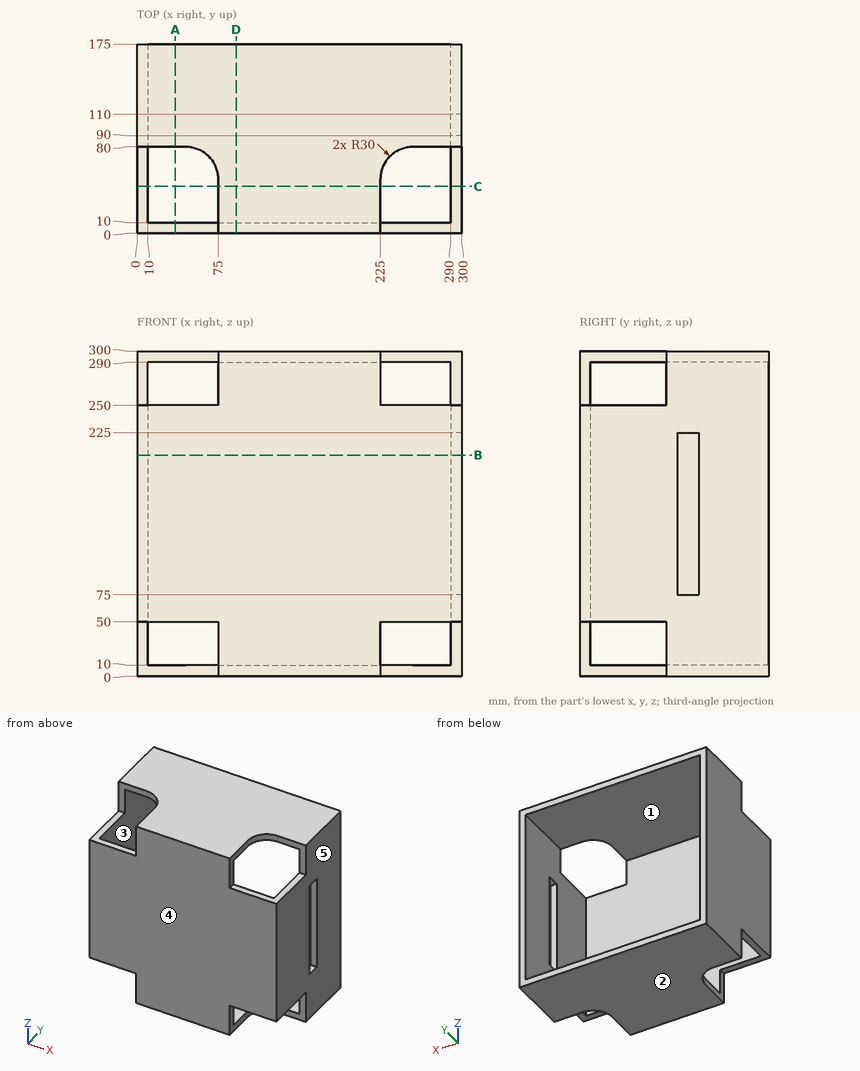
Study the drawing (mm; zero at the part's minimum x, y, z) and answer. A direction names the side the tool comes from. Give positions to 0.01 mm unless a question says otherwise; leave off trailing zeros. Write each loop counter-clockwise with the first axis right and the second up, starting at its lowest first coordinate (ties: lowest second). Pieces come first, ordered by that corner, then holes. Notation, with made-up numbers: (19.5, 22.5) - (42.5, 22.5) arc R23 cw to (42.5, 32.5) - close; hole circle Ø5 at (-35.5, 33.25). An arc over 180 degrees is marked (long way). Write item = value, one per line. Start each with the question number.
Item 1: Each of these flat-tipped pins is pushed along its axis until it touches: P1, Ø13.5, axis at x = 288, z = 25, coming from the -Y side; P2, Ø1, axis at y = 114.5, z = 33.5, coming from the -X side; P3, Ø25, axis at y = 20, z = 16, coming from the -X side; P4, Ø5, axis at x = 136, z = 211, coming from the +Y side. Where does it stop, or does it pass through?
Item 2: Find section B-B (z = 204). Give the vertices of the cut face in (x, y), then the cut area to 3 significant figures.
Item 3: A tool of negligible diameter and unlimited length cuts with its end or side. For the marked faces 1 and 2, from which of +Z, -Z, +X, -X, +Y, -Y can it reach the whole face along a straight path? Write none if from no direction.
Item 4: The mould has two halves that part along X. Classify the marked faces 3, 4 and 5: +X half, -X half, draft (parallel to the pull), parting line (faces both ways), or undercut.
Item 5: Find section A-A (x = 35.5). Give the vertices of the cut face in (y, z).
Item 6: Find the intervals of material crossed by probe 1 along X at (y, z) = (107.5, 34.5); probe 2 along Y at (x, z) = (226, 211.5), in increasing order. Write a range as [from, to].
Item 7: Find section D-D (x = 91.5). Give the vertices of the cut face in (y, z).
Item 8: Find section C-C (y = 43.5). Give the vertices of the cut face in (x, z), then the cut area to 3 significant figures.
Response:
q1.P1 = 80
q1.P2 = 0
q1.P3 = 75
q1.P4 = 10
q2.outline = (0, 0) - (300, 0) - (300, 90) - (290, 90) - (290, 10) - (10, 10) - (10, 175) - (0, 175) - close; (290, 110) - (300, 110) - (300, 175) - (290, 175) - close
q2.area = 6,100 mm²
q3.face_1 = +Y
q3.face_2 = -Z, +X, -X, +Y, -Y
q4.face_3 = undercut
q4.face_4 = draft
q4.face_5 = +X half
q5.outline = (0, 50) - (10, 50) - (10, 250) - (0, 250) - close; (80, 0) - (175, 0) - (175, 10) - (80, 10) - close; (80, 290) - (175, 290) - (175, 300) - (80, 300) - close
q6.probe_1 = [0, 10], [290, 300]
q6.probe_2 = [0, 10]
q7.outline = (0, 0) - (175, 0) - (175, 10) - (10, 10) - (10, 290) - (175, 290) - (175, 300) - (0, 300) - close
q8.outline = (0, 50) - (10, 50) - (10, 250) - (0, 250) - close; (75, 0) - (225, 0) - (225, 10) - (75, 10) - close; (75, 290) - (225, 290) - (225, 300) - (75, 300) - close; (290, 50) - (300, 50) - (300, 250) - (290, 250) - close
q8.area = 7,000 mm²
